Read the model definition and answer for the solid it produces. Units are mm, in the model's axes. A direction names the side the tool comes from. Give positions to 0.01 mm unless a question says otherwise; leave off trailing zeros. Loops run counter-clockwise (first coordinate to the right, second up) from the corner with the lowest first, then second, coordinate; pieces in that order, holes last. Notation, with made-up numbers: (-27, 59) -> (21, 59) arc R20 cw to (21, 65) -> close; hole circle Ø7 at (14.5, 46). An arc over 180 degrees is marked (long way). Write each question's results on one line, items separated by ' | '. Start each with the question number.
Item 1: Section A-A on y = 0 is taken. Write down the section's boundary in (x, z).
Item 2: Which of the six approach directions +Z, -Z, +X, -X, +Y, -Y give full straight-line access (tool end or side, diameter ignored) to faces 1 (the flat face through (41.2, 31.3, 0.1)), 2 (the flat face through (-43, 12.5, 0)), 3 (the flat face through (13, 22, -2))?
Item 3: Section B-B on x = -35 is taken. Write down the section's boundary in (y, z).
Item 4: Section C-C on z = 4 is taken. Write down the section's boundary in (x, y).
Item 5: Find the intervals of material crossed by line 1 (Y direction, x = -35, z = -2.25); line 2 (X direction, y = -13, z = -2.5); line 3 (X direction, y = -6.5, z = 4.75), in increasing order.
Item 6: Section D-D on x = -14.5 is taken. Write down the section's boundary in (y, z), and give its area (3 significant figures).
Item 7: Determine the mould class of faces 4 (the flat face through (37, 18, 3)), 5 (the flat face through (41.3, -31.2, -0.1)), 6 (the flat face through (29.4, 0.5, 5)), 7 (the flat face through (-33, -22, 3)) for opening direction Y: +Y half, -Y half, draft (parallel to the pull), parting line (faces both ways), or undercut.
Item 8: Each of these flat-tipped pins is pushed along its axis until it touches: P1, Ø2.5, axis at x = 42, z = 2, coming from the +Y side; P2, Ø2.5, axis at x = -35, y = -20, coming from the +Z side; P3, Ø1.5, axis at x = -42.5, z = 1.5, coming from the +Y side; P4, Ø4, axis at x = 35.5, y = 20, coming from the +Z side. Where does it stop, or does it pass through?
```python
from build123d import *

# Parameters (mm, degrees)
CROQUIS1_W              = 90
CROQUIS1_H              = 70
CROQUIS1_R              = 28.9
CROQUIS1_R_2            = 2.25
SALIENTE_EXTRUIR1_DEPTH = 5
CROQUIS2_R              = 28.9
CROQUIS2_R_2            = 25
SALIENTE_EXTRUIR2_DEPTH = 3
CROQUIS3_R              = 4.25
CORTAR_EXTRUIR1_DEPTH   = 2
CROQUIS4_W              = 10
CROQUIS4_H              = 25
CORTAR_EXTRUIR2_DEPTH   = 58.879184514
CHAFL_N2_SIZE           = 7.5


with BuildPart() as part:
    # Croquis1 → Saliente-Extruir1 (new, symmetric)
    with BuildSketch(Plane.XY):
        Rectangle(CROQUIS1_W, CROQUIS1_H)
        Circle(CROQUIS1_R, mode=Mode.SUBTRACT)
        with Locations((35, 20)):
            Circle(CROQUIS1_R_2, mode=Mode.SUBTRACT)
        with Locations((35, -20)):
            Circle(CROQUIS1_R_2, mode=Mode.SUBTRACT)
        with Locations((-35, -20)):
            Circle(CROQUIS1_R_2, mode=Mode.SUBTRACT)
        with Locations((-35, 20)):
            Circle(CROQUIS1_R_2, mode=Mode.SUBTRACT)
    extrude(amount=SALIENTE_EXTRUIR1_DEPTH, both=True)

    # Croquis2 → Saliente-Extruir2 (add)
    with BuildSketch(Plane(origin=(0, 0, -5), x_dir=(-1, 0, 0), z_dir=(0, 0, -1))):
        Circle(CROQUIS2_R)
        Circle(CROQUIS2_R_2, mode=Mode.SUBTRACT)
    extrude(amount=-SALIENTE_EXTRUIR2_DEPTH)

    # Croquis3 → Cortar-Extruir1 (cut)
    with BuildSketch(Plane.XY.offset(5)):
        with Locations((-35, 20)):
            Circle(CROQUIS3_R)
        with Locations((35, 20)):
            Circle(CROQUIS3_R)
        with Locations((35, -20)):
            Circle(CROQUIS3_R)
        with Locations((-35, -20)):
            Circle(CROQUIS3_R)
    extrude(amount=-CORTAR_EXTRUIR1_DEPTH, mode=Mode.SUBTRACT)

    # Croquis4 → Cortar-Extruir2 (cut, through all)
    with BuildSketch(Plane.XY.offset(5)):
        with Locations((-45, 0)):
            Rectangle(CROQUIS4_W, CROQUIS4_H)
        with Locations((45, 0)):
            Rectangle(CROQUIS4_W, CROQUIS4_H)
    extrude(amount=-CORTAR_EXTRUIR2_DEPTH, mode=Mode.SUBTRACT)

    # Chaflán2
    chafl_n2_edges = [part.edges().sort_by_distance(p)[0] for p in [
        (45, -35, 0),
        (-45, -35, 0),
        (-45, 35, 0),
        (45, 35, 0),
    ]]
    chamfer(chafl_n2_edges, length=CHAFL_N2_SIZE)


solid = part.part
```
Findings:
1) outline: (-40, -5) -> (-25, -5) -> (-25, -2) -> (-28.9, -2) -> (-28.9, 5) -> (-40, 5) -> close; (25, -5) -> (40, -5) -> (40, 5) -> (28.9, 5) -> (28.9, -2) -> (25, -2) -> close
2) face 1: +Z, -Z, +X, +Y | face 2: +Z, -Z, -X | face 3: +Z
3) outline: (-35, -5) -> (-22.25, -5) -> (-22.25, 3) -> (-24.25, 3) -> (-24.25, 5) -> (-35, 5) -> close; (-17.75, -5) -> (17.75, -5) -> (17.75, 3) -> (15.75, 3) -> (15.75, 5) -> (-15.75, 5) -> (-15.75, 3) -> (-17.75, 3) -> close; (22.25, -5) -> (35, -5) -> (35, 5) -> (24.25, 5) -> (24.25, 3) -> (22.25, 3) -> close
4) outline: (-45, -27.5) -> (-37.5, -35) -> (37.5, -35) -> (45, -27.5) -> (45, -12.5) -> (40, -12.5) -> (40, 12.5) -> (45, 12.5) -> (45, 27.5) -> (37.5, 35) -> (-37.5, 35) -> (-45, 27.5) -> (-45, 12.5) -> (-40, 12.5) -> (-40, -12.5) -> (-45, -12.5) -> close; hole circle Ø8.5 at (-35, -20); hole circle Ø8.5 at (-35, 20); hole circle Ø57.8 at (0, 0); hole circle Ø8.5 at (35, -20); hole circle Ø8.5 at (35, 20)
5) line 1: -35 to -22.25, -17.75 to 17.75, 22.25 to 35 | line 2: -45 to -21.35, 21.35 to 45 | line 3: -40 to -28.16, 28.16 to 40
6) outline: (-35, -5) -> (-20.37, -5) -> (-20.37, -2) -> (-25, -2) -> (-25, 5) -> (-35, 5) -> close; (20.37, -5) -> (35, -5) -> (35, 5) -> (25, 5) -> (25, -2) -> (20.37, -2) -> close | area: 228 mm2
7) face 4: undercut | face 5: -Y half | face 6: draft | face 7: undercut
8) P1: y = 31.75 | P2: through | P3: y = 30.75 | P4: z = 3
